Autodesk Inventor part; units mm, degrees
ref_plane "YZ Plane" through (0, 0, 0) normal (1, 0, 0) x (0, 1, 0)
ref_plane "XZ Plane" through (0, 0, 0) normal (0, 1, 0) x (-1, 0, 0)
ref_plane "XY Plane" through (0, 0, 0) normal (0, 0, 1) x (1, 0, 0)
sketch "Sketch1" plane through (0, 0, 0) normal (0, 1, 0) x (-1, 0, 0)
  line L0 (0, 0) -> (25, 0)
  line L1 (25, 0) -> (25, -90)
  line L2 (25, -90) -> (0, -90)
  line L3 (0, -90) -> (0, 0)
  dimension "d0" = 25
  dimension "d1" = 90
extrude "Extrusion1" add sketch "Sketch1" along normal blind 10
sketch "Sketch2" plane through (0, 10, 0) normal (0, 1, 0) x (1, 0, 0)
  line L0 (-25, 90) -> (-25, 0)
  line L1 (0, 0) -> (0, 90)
  line L2 (-25, 37.5) -> (0, 37.5)
  line L3 (0, 37.5) -> (0, 52.5)
  line L4 (0, 52.5) -> (-25, 52.5)
  line L5 (-25, 52.5) -> (-25, 37.5)
  line L6 (-25, 0) -> (0, 0)
  point P0 (-25, 80)
  point P1 (-25, 10)
  point P2 (0, 10)
  point P3 (0, 80)
  point P4 (-15, 0)
  point P5 (-10, 0)
  point P6 (0, 37.5)
  dimension "d5" = 15
  dimension "d6" = 37.5
extrude "Extrusion2" add sketch "Sketch2" along normal blind 22 contours L4 L1 L2 L0
sketch "Sketch3" plane through (-25, 10, -37.5) normal (0, 0, 1) x (1, 0, 0)
  point P0 (25, -10)
sketch "Sketch5" plane through (0, 0, 0) normal (1, 0, 0) x (0, 0, -1)
  line L0 (37.5, 10) -> (37.5, 32)
  line L1 (0, 10) -> (37.5, 10)
  line L2 (37.5, 32) -> (0, 10)
  line L3 (37.5, 32) -> (52.5, 32)
  line L4 (52.5, 32) -> (90, 10)
  line L5 (90, 10) -> (52.5, 10)
  line L6 (52.5, 10) -> (90, 10)
  line L7 (52.5, 10) -> (52.5, 32)
  line L8 (52.5, 32) -> (52.5, 10)
  point P0 (0, 0)
extrude "Extrusion3" add sketch "Sketch5" against normal blind 25
fillet "Fillet2" radius 10 4 edges at (-25, 5, 0) (0, 5, 0) (-25, 5, -90) (0, 5, -90)
fillet "Fillet3" radius 2 14 edges at (-12.5, 32, -52.5) (-12.5, 32, -37.5) (0, 32, -45) (-2.9289, 11.7183, -87.0711) (-12.5, 10, -90) (-22.0711, 11.7183, -87.0711) (-25, 23.9333, -66.25) (0, 23.9333, -66.25) (-2.9289, 11.7183, -2.9289) (-12.5, 10, 0) (-22.0711, 11.7183, -2.9289) (-25, 23.9333, -23.75) (0, 23.9333, -23.75) (-25, 32, -45)
sketch "Sketch6" plane through (-25, 0, -80) normal (-1, 0, 0) x (0, 0, 1)
  line L0 (28.0434, 30) -> (41.9566, 30)
  line L1 (35, 30) -> (35, 15)
  line L2 (70, 0) -> (0, 0)
  line L3 (35, 30) -> (35, 0)
  line L4 (35, 15) -> (35, 0)
  circle A0 centre (35, 7.5) radius 3
  point P0 (80, 0)
  point P1 (35, 22.5)
  dimension "d13" = 6
  dimension "d14" = 7.5
extrude "Extrusion4" cut sketch "Sketch6" against normal blind 25
sketch "Sketch7" plane through (-25, 0, -80) normal (-1, 0, 0) x (0, 0, 1)
  line L0 (35, 25.5581) -> (35, 19.5581)
  circle A0 centre (35, 7.5) radius 3
  line L1 (35, 10.5) -> (35, 4.5)
  circle A1 centre (35, 7.5) radius 5
  point P0 (80, 0)
  point P1 (35, 22.5581)
  dimension "d19" = 10
extrude "Extrusion5" cut sketch "Sketch7" against normal blind 10
fillet "Fillet4" radius 1 1 edges at (-25, 7.5, -50)
sketch "Sketch8" plane through (0, 0, 0) normal (0, -1, 0) x (1, 0, 0)
  line L0 (-10, -90) -> (-15, -90)
  line L1 (-12.5, -90) -> (-12.5, 0)
  line L2 (-15, 0) -> (-10, 0)
  circle A0 centre (-12.5, -80.5935) radius 5
  circle A1 centre (-12.5, -9.4065) radius 5
  point P0 (0, 0)
  point P1 (-12.5, -45)
  point P2 (-12.5, -4.4065)
  point P3 (-12.5, -14.4065)
  point P4 (-12.5, -75.5935)
  point P5 (-12.5, -85.5935)
  dimension "d23" = 71.187
  dimension "d24" = 10
  dimension "d25" = 10
  dimension "d26" = 35.5935
extrude "Extrusion6" cut sketch "Sketch8" against normal blind 10
properties part number "Triangle_Bracket"
Model file for the job. Use its own axes, mm. A direction names the side the tool comes from. Coordinates: 2 decimals unless noted, no trailing zeros. Write each loop counter-clockwise with the first axis right and the second up, starting at its lowest first coordinate (ties: lowest second). Pieces come first, ordered by that corner, then holes. Notation, with made-up numbers: (1, -12.75) - (17, -12.75) arc R35 cw to (17, 26.25) - close; hole circle Ø8 at (-11, 55.25). An arc over 180 degrees is marked (long way). Use a Markdown table: item, result. Add a question column.
Item 1: Drill centre lines: line 1 along Z through (x, y) = (-12.5, 7.75); line 2 along Y through (x, z) = (-19.25, -45); line 3 along Z through (x, y) = (-13.25, 7). Where is each one in solid material? Low to high.
Item 2: Band-saw the part on B-B, the plane y = 7.5. Write the cut outline in (x, z).
Item 3: Band-saw the part on A-A, the plane z = -45. Write the cut outline in (x, y).
Item 4: 3-axis set-ups, long thin cutter, end or side, ignore diameter. For faces 1 (the face through (-12.53, 9.86, -89.73)), 2 (the face through (-19.563, 7.72, -49.995)), 3 (the face through (-13, 10, -81)): which of +Z, -Z, +X, -X, +Y, -Y reach the whole face in a straight line?
Item 5: Drop flat-ended pins along their axis: pin 1 (1 mm diameter, centred on y = 7.5, z = -63, fed in from +X); pin 2 (3 mm diameter, centred on x = -21, y = 26.5, fed in from -Z); pin 3 (8 mm diameter, centred on x = -12.5, z = -9.41, fed in from -Y); pin 4 (6 mm diameter, centred on x = -13.5, z = -68, fed in from +Y). Give the stop position or say it passes through.
Item 6: Two-plate mould, pull along X, no slides. Class faces 4 (the face through (-21.99, 5.36, -87.15)), 5 (the face through (-13, 4, -90)), 6 (the face through (-7.73, 4.93, -79.09)): pulls with the +X half, pulls with the -X half, needs draft (parallel to the pull), parting line crosses it, or undercut.
A:
| question | item | result |
|---|---|---|
| 1 | line 1 | z = -90 to -85.59, -75.59 to -47.99, -42.01 to -14.41, -4.41 to 0 |
| 1 | line 2 | y = 0 to 2.5, 12.5 to 32 |
| 1 | line 3 | z = -90 to -85.54, -75.65 to -47.96, -42.04 to -14.35, -4.46 to 0 |
| 2 | outline | (-25, -80) arc R10 ccw to (-15, -90) - (-10, -90) arc R10 ccw to (0, -80) - (0, -48) - (-15, -48) - (-15, -50) - (-24, -50) arc R1 ccw to (-25, -51) - close; (-25, -39) arc R1 ccw to (-24, -40) - (-15, -40) - (-15, -42) - (0, -42) - (0, -10) arc R10 ccw to (-10, 0) - (-15, 0) arc R10 ccw to (-25, -10) - close; hole circle Ø10 at (-12.5, -80.59); hole circle Ø10 at (-12.5, -9.41) |
| 3 | outline | (-25, 0) - (0, 0) - (0, 4.5) - (-15, 4.5) - (-15, 2.5) - (-24, 2.5) arc R1 ccw to (-25, 1.5) - close; (-25, 13.5) arc R1 ccw to (-24, 12.5) - (-15, 12.5) - (-15, 10.5) - (0, 10.5) - (0, 30) arc R2 ccw to (-2, 32) - (-23, 32) arc R2 ccw to (-25, 30) - close |
| 4 | face 1 | -Z, +X, -X, +Y |
| 4 | face 2 | -X |
| 4 | face 3 | -Y |
| 5 | pin 1 | stops at x = 0 |
| 5 | pin 2 | stops at z = -64.43 |
| 5 | pin 3 | stops at y = 10 |
| 5 | pin 4 | stops at y = 24.67 |
| 6 | face 4 | pulls with the -X half |
| 6 | face 5 | needs draft |
| 6 | face 6 | undercut |
